from build123d import *

# Parameters (mm, degrees)
F1_DEPTH     = 254
F2_T1_DEPTH  = 254
F2_T3_DEPTH  = 203.2
F2_T5_DEPTH  = 179.07
F2_T7_DEPTH  = 279.4
F2_T9_DEPTH  = 154.94
F2_T11_DEPTH = 203.2
F2_T14_ANGLE = 90
F2_T16_ANGLE = 90
F2_T18_ANGLE = 90
F2_T20_ANGLE = 90
F3_R         = 4.0000047
F3_R_2       = 1.5875
F4_DEPTH     = 203.2


# Not quite as in the source:
# - a fillet or chamfer that OpenCascade refuses, or shapes differently, is made with other operations: its cross-section is extruded or revolved along the edge and cut away or added


with BuildPart() as f1:
    # F0 (on Front) → F1 (new body)
    with BuildSketch(Plane.XZ):
        Polygon((-88.9, -88.9), (88.9, -88.9), (88.9, 88.9), (82.55, 88.9), (82.55, -82.55), (-82.55, -82.55), (-82.55, 88.9), (-88.9, 88.9), align=None)
    extrude(amount=F1_DEPTH)

    # F2: fillet of radius 5.08 on 11 edges, made by hand

    # F2_s2 → F2_t1 (join)
    with BuildSketch(Plane.XZ):
        with BuildLine():
            ThreePointArc((82.55, -77.47), (81.0621024484, -81.0621024484), (77.47, -82.55))
            Line((77.47, -82.55), (82.55, -82.55))
            Line((82.55, -82.55), (82.55, -77.47))
        make_face()
        with BuildLine():
            ThreePointArc((-77.47, -82.55), (-81.0621024484, -81.0621024484), (-82.55, -77.47))
            Line((-82.55, -77.47), (-82.55, -82.55))
            Line((-82.55, -82.55), (-77.47, -82.55))
        make_face()
    extrude(amount=F2_T1_DEPTH)

    # F2_s4 → F2_t3 (cut)
    with BuildSketch(Plane.YZ.offset(-101.6)):
        with BuildLine():
            ThreePointArc((-254, -83.82), (-252.5121024484, -87.4121024484), (-248.92, -88.9))
            Line((-248.92, -88.9), (-254, -88.9))
            Line((-254, -88.9), (-254, -83.82))
        make_face()
    extrude(amount=F2_T3_DEPTH, mode=Mode.SUBTRACT)

    # F2_s6 → F2_t5 (cut)
    with BuildSketch(Plane.XY.offset(-77.47)):
        with BuildLine():
            ThreePointArc((-82.55, -248.92), (-84.0378975516, -252.5121024484), (-87.63, -254))
            Line((-87.63, -254), (-82.55, -254))
            Line((-82.55, -254), (-82.55, -248.92))
        make_face()
        with BuildLine():
            ThreePointArc((87.63, 0), (84.0378975516, -1.4878975516), (82.55, -5.08))
            Line((82.55, -5.08), (82.55, 0))
            Line((82.55, 0), (87.63, 0))
        make_face()
        with BuildLine():
            ThreePointArc((87.63, -254), (84.0378975516, -252.5121024484), (82.55, -248.92))
            Line((82.55, -248.92), (82.55, -254))
            Line((82.55, -254), (87.63, -254))
        make_face()
        with BuildLine():
            ThreePointArc((-82.55, -5.08), (-84.0378975516, -1.4878975516), (-87.63, 0))
            Line((-87.63, 0), (-82.55, 0))
            Line((-82.55, 0), (-82.55, -5.08))
        make_face()
    extrude(amount=F2_T5_DEPTH, mode=Mode.SUBTRACT)

    # F2_s8 → F2_t7 (cut)
    with BuildSketch(Plane.XZ.offset(-12.7)):
        with BuildLine():
            ThreePointArc((87.63, 88.9), (84.0378975516, 87.4121024484), (82.55, 83.82))
            Line((82.55, 83.82), (82.55, 88.9))
            Line((82.55, 88.9), (87.63, 88.9))
        make_face()
    extrude(amount=F2_T7_DEPTH, mode=Mode.SUBTRACT)

    # F2_s10 → F2_t9 (cut)
    with BuildSketch(Plane.YZ.offset(-77.47)):
        with BuildLine():
            ThreePointArc((0, -87.63), (-1.4878975516, -84.0378975516), (-5.08, -82.55))
            Line((-5.08, -82.55), (0, -82.55))
            Line((0, -82.55), (0, -87.63))
        make_face()
        with BuildLine():
            ThreePointArc((-254, -87.63), (-252.5121024484, -84.0378975516), (-248.92, -82.55))
            Line((-248.92, -82.55), (-254, -82.55))
            Line((-254, -82.55), (-254, -87.63))
        make_face()
    extrude(amount=F2_T9_DEPTH, mode=Mode.SUBTRACT)

    # F2_s12 → F2_t11 (cut)
    with BuildSketch(Plane.XY.offset(-101.6)):
        with BuildLine():
            ThreePointArc((-88.9, -248.92), (-87.4121024484, -252.5121024484), (-83.82, -254))
            Line((-83.82, -254), (-88.9, -254))
            Line((-88.9, -254), (-88.9, -248.92))
        make_face()
    extrude(amount=F2_T11_DEPTH, mode=Mode.SUBTRACT)

    # F2_s13 → F2_t14 (revolve, cut)
    with BuildSketch(Plane.YZ.offset(-77.47)):
        with BuildLine():
            ThreePointArc((0, -87.63), (-1.4878975516, -84.0378975516), (-5.08, -82.55))
            Line((-5.08, -82.55), (0, -82.55))
            Line((0, -82.55), (0, -87.63))
        make_face()
    revolve(axis=Axis((-77.47, 0, -77.47), (0, 1, 0)), revolution_arc=F2_T14_ANGLE, mode=Mode.SUBTRACT)

    # F2_s15 → F2_t16 (revolve, cut)
    with BuildSketch(Plane.XY.offset(-77.47)):
        with BuildLine():
            ThreePointArc((87.63, -254), (84.0378975516, -252.5121024484), (82.55, -248.92))
            Line((82.55, -248.92), (82.55, -254))
            Line((82.55, -254), (87.63, -254))
        make_face()
    revolve(axis=Axis((77.47, -254, -77.47), (0, 1, 0)), revolution_arc=F2_T16_ANGLE, mode=Mode.SUBTRACT)

    # F2_s17 → F2_t18 (revolve, cut)
    with BuildSketch(Plane.YZ.offset(-77.47)):
        with BuildLine():
            ThreePointArc((-254, -87.63), (-252.5121024484, -84.0378975516), (-248.92, -82.55))
            Line((-248.92, -82.55), (-254, -82.55))
            Line((-254, -82.55), (-254, -87.63))
        make_face()
    revolve(axis=Axis((-77.47, -254, -77.47), (0, 1, 0)), revolution_arc=F2_T18_ANGLE, mode=Mode.SUBTRACT)

    # F2_s19 → F2_t20 (revolve, cut)
    with BuildSketch(Plane.XY.offset(-77.47)):
        with BuildLine():
            ThreePointArc((87.63, 0), (84.0378975516, -1.4878975516), (82.55, -5.08))
            Line((82.55, -5.08), (82.55, 0))
            Line((82.55, 0), (87.63, 0))
        make_face()
    revolve(axis=Axis((77.47, 0, -77.47), (0, 1, 0)), revolution_arc=F2_T20_ANGLE, mode=Mode.SUBTRACT)

    # F3 (on face) → F4 (cut)
    with BuildSketch(Plane(origin=(-88.9, 0, 0), x_dir=(0, -1, 0), z_dir=(-1, 0, 0))):
        with Locations((203.2, 50.8)):
            Circle(F3_R)
        with Locations((211.328, 50.8)):
            Circle(F3_R_2)
        with Locations((203.2, 42.672)):
            Circle(F3_R_2)
        with Locations((195.072, 50.8)):
            Circle(F3_R_2)
        with Locations((203.2, 58.928)):
            Circle(F3_R_2)
    extrude(amount=-F4_DEPTH, mode=Mode.SUBTRACT)


solid = f1.part
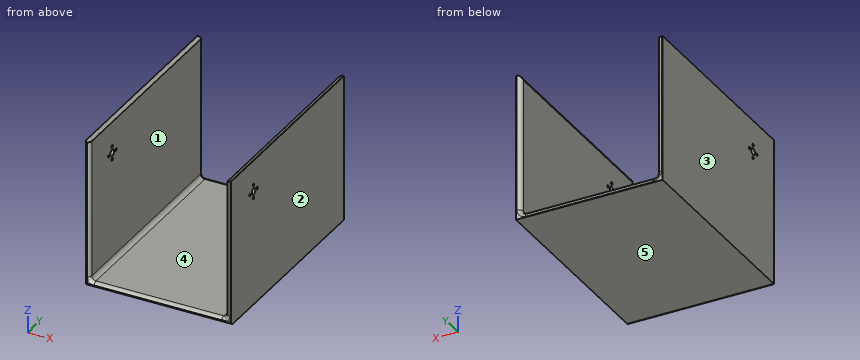
The model under review builds one solid part; all positions refer to its coordinate system, in mm. Face numbers are marked on the shaded views. A direction names the side the tool comes from. Give positions to 0.01 mm unless a question says otherwise; leave off trailing zeros. Loops run counter-clockwise (first coordinate to the right, second up) from the corner with the lowest first, then second, coordinate; pieces in that order, holes last. Notation, with made-up numbers: (80.5, 56) -> (95.5, 56) arc R14 ccw to (95.5, 74) -> close; hole circle Ø7 at (48, 79.25). An arc over 180 degrees is marked (long way). Put each result on its own line as item: value. Start each with the question number.
1. Mouldability with a two-part tool opening along X and no side actions: class the marked faces 1, 2 and 3 as released by +X, released by -X, zero draft, split by the parting line, or undercut.
2. We need section B-B on y = -165.5. State the section outline as (x, z) points.
3. Wall thickness on probe 1 along Z at (x, y) = (-85.5, -203.2); probe 2 along X at (y, z) = (-125.5, 81.5): over which ranges is each line inside the solid? List them lowest first.
4. We need section A-A on z = -47. State the section outline as (x, y) points (3 decimals).
5. Clearance check with flat-ended pins moving along their axes: P1, Ø1.9, axis at y = -203.2, z = 42.672, coming from the +X side; P2, Ø13, axis at y = -203.2, z = 50.8, coming from the -X side; P3, Ø2, axis at x = -53.5, y = -176.5, coming from the +Z side; P4, Ø1, axis at x = 36, y = -39.5, coming from the +Z side. State where each tip first meets the part, or that it passes through.
6. For the marked faces 4 and 5, list the 3-axis set-ups (+Z, -Z, +X, -X, +Y, -Y) from which the entire face can be reached by the end or side of a thin tool; tool diameter is ignored.
7. We need section C-C on x = -45.5. State the section outline as (y, z) points (3 decimals).
Determined:
1. face 1: undercut
1. face 2: released by +X
1. face 3: released by -X
2. outline: (-88.9, -88.9) -> (88.9, -88.9) -> (88.9, 88.9) -> (87.63, 88.9) arc R5.08 ccw to (82.55, 83.82) -> (82.55, -77.47) arc R5.08 cw to (77.47, -82.55) -> (-77.47, -82.55) arc R5.08 cw to (-82.55, -77.47) -> (-82.55, 88.9) -> (-88.9, 88.9) -> close
3. probe 1: -88.9 to 41.08, 44.26 to 46.8, 54.8 to 57.34, 60.52 to 88.9
3. probe 2: -88.9 to -82.55, 82.55 to 88.9
4. outline: (-88.9, -248.92) arc R5.08 ccw to (-85.725, -253.629) arc R5.08 ccw to (-82.55, -248.92) -> (-82.55, -5.08) arc R5.08 ccw to (-87.63, 0) -> (-88.9, 0) -> close; (82.55, -248.92) arc R5.08 ccw to (87.63, -254) -> (88.9, -254) -> (88.9, 0) -> (87.63, 0) arc R5.08 ccw to (82.55, -5.08) -> close
5. P1: through
5. P2: x = -88.9
5. P3: z = -82.55
5. P4: z = -82.55
6. face 4: +Z, +Y, -Y
6. face 5: -Z, +X, -X, +Y, -Y
7. outline: (-253.629, -85.725) arc R5.08 ccw to (-248.92, -88.9) -> (0, -88.9) -> (0, -87.63) arc R5.08 ccw to (-5.08, -82.55) -> (-248.92, -82.55) arc R5.08 ccw to start
